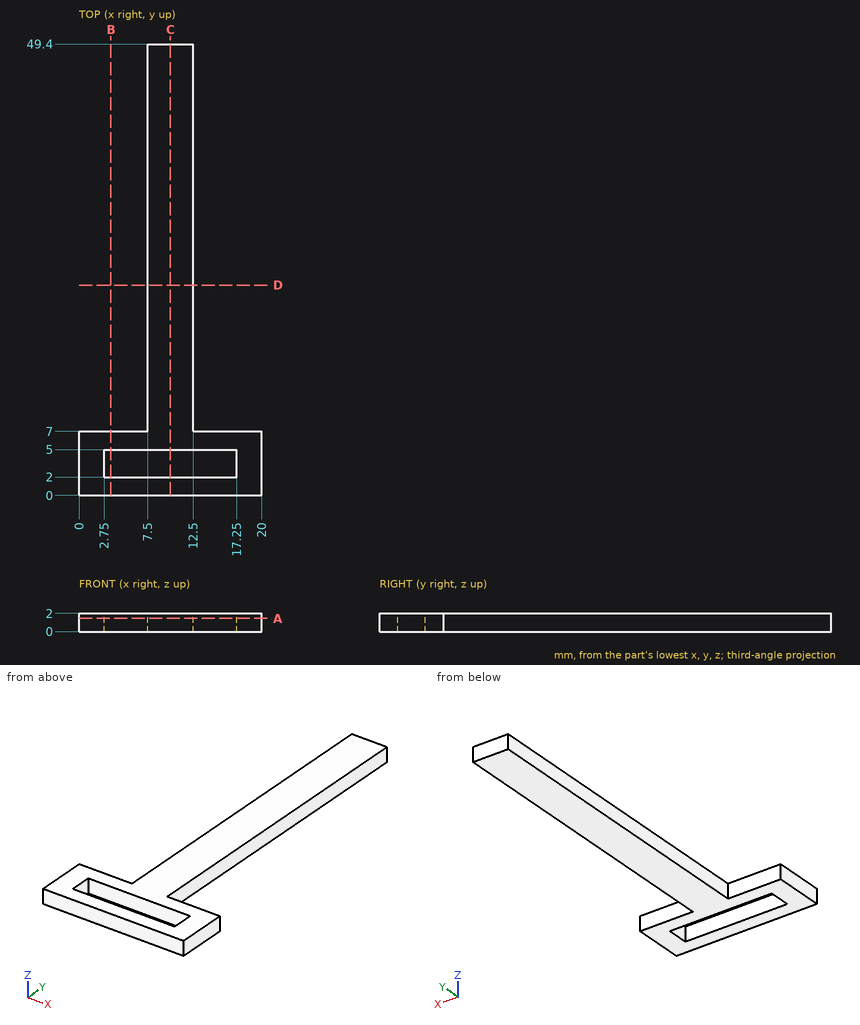
Source: three-view drawing plus pictorial views. Frame: mm from the lowest corner of the part. Round coordinates to 2 decimals unless told otherwise and drop trailing zeros. Loops run counter-clockwise (first coordinate to the right, second up) from the corner with the lowest first, then second, coordinate; pieces in that order, holes last.
Item 1: Section A-A, the plane z = 1.45. Output: boundary loops of the cut face in (x, y).
Checked values:
outline: (0, 0) - (20, 0) - (20, 7) - (12.5, 7) - (12.5, 49.4) - (7.5, 49.4) - (7.5, 7) - (0, 7) - close; hole (2.75, 2) - (17.25, 2) - (17.25, 5) - (2.75, 5) - close
Item 2: Section D-D, the plane y = 23. Output: boundary loops of the cut face in (x, z).
Checked values:
outline: (7.5, 0) - (12.5, 0) - (12.5, 2) - (7.5, 2) - close
Item 3: Contact query for flat-ended pins moving along their axis: P1, Ø0.6, axis at y = 25.5, z = 1, coming from the -X side; P2, Ø5, axis at x = 6.5, y = 17, coming from the +Z side; P3, Ø0.6, axis at y = 20.5, z = 1.5, coming from the +X side; P4, Ø1, axis at x = 6.5, y = 12, coming from the +Z side. Output: stop coordinate, or through.
Checked values:
P1: stops at x = 7.5
P2: stops at z = 2
P3: stops at x = 12.5
P4: passes through
Item 4: Section B-B, the plane x = 3.5. Output: boundary loops of the cut face in (y, z).
Checked values:
outline: (0, 0) - (2, 0) - (2, 2) - (0, 2) - close; (5, 0) - (7, 0) - (7, 2) - (5, 2) - close
Item 5: Section C-C, the plane x = 10. Output: boundary loops of the cut face in (y, z).
Checked values:
outline: (0, 0) - (2, 0) - (2, 2) - (0, 2) - close; (5, 0) - (49.4, 0) - (49.4, 2) - (5, 2) - close
Item 6: Line query: L1, parallel to Y at x = 9.75, z = 1.75; L2, parallel to X at y = 3, z = 0.2; L3, parallel to Y at x = 13.25, z = 1.65. Output: solid intervals per line, ascending.
Checked values:
L1: y = 0 to 2, 5 to 49.4
L2: x = 0 to 2.75, 17.25 to 20
L3: y = 0 to 2, 5 to 7
